from build123d import *

# Parameters (mm, degrees)
EXTRUSION1_DEPTH = 27
ESQUISSE2_R      = 16.7
EXTRUSION2_DEPTH = 37
ESQUISSE3_R      = 5.5
EXTRUSION3_DEPTH = 1.5
ESQUISSE4_R      = 1.35
EXTRUSION4_DEPTH = 10
EXTRUSION5_START = 1.5
ESQUISSE5_R      = 5.5
EXTRUSION5_DEPTH = 1.5
ESQUISSE6_R      = 2
EXTRUSION6_DEPTH = 8.5


with BuildPart() as part:
    # Esquisse1 → Extrusion1 (new body)
    with BuildSketch(Plane.XY):
        with BuildLine():
            Line((-21.263539738, 17.051170213), (11.736460262, 17.051170213))
            ThreePointArc((11.736460262, 17.051170213), (13.857780605, 16.172490556), (14.736460262, 14.051170213))
            Line((14.736460262, 14.051170213), (14.736460262, -18.948829787))
            ThreePointArc((14.736460262, -18.948829787), (13.857780605, -21.070150131), (11.736460262, -21.948829787))
            Line((11.736460262, -21.948829787), (-21.263539738, -21.948829787))
            ThreePointArc((-21.263539738, -21.948829787), (-23.384860082, -21.070150131), (-24.263539738, -18.948829787))
            Line((-24.263539738, -18.948829787), (-24.263539738, 14.051170213))
            ThreePointArc((-24.263539738, 14.051170213), (-23.384860082, 16.172490556), (-21.263539738, 17.051170213))
        make_face()
    extrude(amount=EXTRUSION1_DEPTH)

    # Esquisse2 → Extrusion2 (add)
    with BuildSketch(Plane.XY.offset(27)):
        with Locations(Location((-4.763539738, -2.448829787, 0), (0, 0, 180))):
            Circle(ESQUISSE2_R)
    extrude(amount=EXTRUSION2_DEPTH)

    # Esquisse3 → Extrusion3 (add)
    with BuildSketch(Plane.XY.offset(64)):
        with Locations((-4.763539738, -2.448829787)):
            Circle(ESQUISSE3_R)
    extrude(amount=EXTRUSION3_DEPTH)

    # Esquisse4 → Extrusion4 (cut)
    with BuildSketch(Plane(origin=(0, 0, 0), x_dir=(-1, 0, 0), z_dir=(0, 0, -1))):
        with Locations((-11.236460262, 13.551170213)):
            Circle(ESQUISSE4_R)
        with Locations((20.763539738, 13.551170213)):
            Circle(ESQUISSE4_R)
        with Locations((20.763539738, -18.448829787)):
            Circle(ESQUISSE4_R)
        with Locations((-11.236460262, -18.448829787)):
            Circle(ESQUISSE4_R)
    extrude(amount=-EXTRUSION4_DEPTH, mode=Mode.SUBTRACT)

    # Esquisse5 → Extrusion5 (add)
    with BuildSketch(Plane(origin=(0, 0, 0), x_dir=(-1, 0, 0), z_dir=(0, 0, -1)).offset(EXTRUSION5_START)):
        with Locations(Location((4.763539738, -2.448829787, 0), (0, 0, 180))):
            Circle(ESQUISSE5_R)
    extrude(amount=-EXTRUSION5_DEPTH)

    # Esquisse6 → Extrusion6 (add)
    with BuildSketch(Plane(origin=(0, 0, -1.5), x_dir=(-1, 0, 0), z_dir=(0, 0, -1))):
        with Locations((4.763539738, -2.448829787)):
            Circle(ESQUISSE6_R)
    extrude(amount=EXTRUSION6_DEPTH)


solid = part.part
Design review of the part built by this model. Coordinates are the model's own, in mm. A direction names the side the tool comes from. Give positions to 0.01 mm unless a question says otherwise; leave off trailing zeros. Write each loop counter-clockwise with the first axis right and the second up, starting at its lowest first coordinate (ties: lowest second). Pieces come first, ordered by that corner, then holes. Notation, with made-up numbers: M -30,16.25 L -2,16.25 A35 cw -2,51.25 Z; hole C 5.5,32.25 d1. An arc over 180 degrees is marked long. Return JSON: item names as keys, results as strings. Group by question number.
Item 1: Take a section at D-D (x = 9). Give the boundary of the cut face in (y, z).
Item 2: Tool access review of faces 1 (the flat face through (-5, -21.949, 13)), 2 (the flat face through (0, 2, 0)), 3 (the flat face through (13, -2, 27)): name each direction out of +Z, -Z, +X, -X, +Y, -Y from which nothing blocks a thin tool from reaching the whole face with its end or side.
Item 3: Clearance check with flat-ended pins moving along their axes: pin 1 Ø5 at (x, z) = (-3.5, 39) entering from -Y; pin 2 Ø0.8 at (x, y) = (12, 13.5) entering from -Z; pin 3 Ø1 at (x, z) = (-2, 34) entering from -Y. State where each tip first meets the part, or that it passes through.
Item 4: Take a section at C-C (z = 33). Give the boundary of the cut face in (x, y), plus the area to 3 significant figures.
Item 5: The part is to be moulded in two halves that separate along Y. For faces 4 (the cylindrical face through (-20.471, 12.233, 4.93)), 5 (the flat face through (-5, -2, -10)), 6 (the cylindrical face through (13.83, 16.2, 13.31)), say which applies: pulls with the +Y half, pulls with the -Y half, needs draft (parallel to the pull), parting line crosses it, or undercut.
Item 6: Take a section at B-B (y = -12). Give the boundary of the cut face in (x, z).
Item 7: Take a section at A-A (x = -8.5). Give the boundary of the cut face in (y, z).
Item 8: Wall thickness on line 1 along Z through (x, y) = (-10, -19.5); line 2 along Y through (x, z) = (-5.5, 58); line 3 along Y through (x, z) = (-21.5, 21): over which ranges is each line inside the solid? List them lowest first.
Return value:
{
 "1": {"outline": "M -21.95,0 L 17.05,0 L 17.05,27 L 7.01,27 L 7.01,64 L -11.91,64 L -11.91,27 L -21.95,27 Z"},
 "2": {"face 1": "+Z, -Z, +X, -X, -Y", "face 2": "-Z", "face 3": "+Z"},
 "3": {"pin 1": "stops at y = -19.15", "pin 2": "stops at z = 10", "pin 3": "stops at y = -18.99"},
 "4": {"outline": "C -4.76,-2.45 d33.4", "area": "876 mm2"},
 "5": {"face 4": "undercut", "face 5": "needs draft", "face 6": "pulls with the +Y half"},
 "6": {"outline": "M -24.26,0 L 14.74,0 L 14.74,27 L 8.94,27 L 8.94,64 L -18.46,64 L -18.46,27 L -24.26,27 Z"},
 "7": {"outline": "M -21.95,0 L -6.48,0 L -6.48,-1.5 L 1.59,-1.5 L 1.59,0 L 17.05,0 L 17.05,27 L 13.83,27 L 13.83,64 L 1.59,64 L 1.59,65.5 L -6.48,65.5 L -6.48,64 L -18.73,64 L -18.73,27 L -21.95,27 Z"},
 "8": {"line 1": "z = 0 to 27", "line 2": "y = -19.13 to 14.23", "line 3": "y = -21.94 to 17.04"}
}
